Design review of the part built by this model. Coordinates are the model's own, in mm. A direction names the side the tool comes from. Coordinates: 2 decimals unless noted, no trailing zeros. Loops run counter-clockwise (first coordinate to the right, second up) from the corner with the lowest first, then second, coordinate; pieces in that order, holes last.
Q1. Add section B-B on z = 19.5. Give the boundary of the cut face in (x, y).
Q2. Wall thickness on probe 1 along Y at (x, z) = (26.5, 10.5); probe 2 along X at (y, z) = (-26.5, 14); probe 3 along Y at (x, z) = (-19, 2): over which ranges is each line inside the solid? List them lowest first.
Q3. Add section A-A on y = 26. Give the boundary of the cut face in (x, z).
Q4. Draft analysis for pull direction X (two halves, no side actions). For faces 3 (the face through (-23.38, -6.41, 12.52)), 4 (the face through (-1, 1, 25.4)), state which applies: released by +X, released by -X, zero draft, split by the parting line, or undercut.
Q5. Machinability: for faces 1 (the face through (17.24, -17.04, 12.52)), 2 (the face through (-1, 1, 0)), which of the approach directions +Z, -Z, +X, -X, +Y, -Y give a long, thin tool a straight path to every point of the face, cutting with its end or side? Answer none if there is none.
Q6. Add section D-D on y = -30. Give the boundary of the cut face in (x, z), and give its area (3 significant figures).
Q7. Add section C-C on x = 2. Give the boundary of the cut face in (y, z), and give its area (3 significant figures).
Q8. For P1, Ø5, axis at x = 20, z = 8, coming from the -Y side; P2, Ø10, axis at y = 16.5, z = 7.5, coming from the -X side; P3, Ø1.5, axis at y = 26, z = 9, coming from the +X side, all flat-tipped, find the tip position at first contact; note any pin that passes through.
```python
from build123d import *

# Parameters (mm, degrees)
F0_R     = 12.7
F1_DEPTH = 25.4


with BuildPart() as f1:
    # F0 (on Top) → F1 (new body)
    with BuildSketch(Plane.XY):
        with BuildLine():
            Line((7.3707728384, 23.1299660417), (4.863097807, 23.7839000386))
            ThreePointArc((4.863097807, 23.7839000386), (-4.0567226722, 14.7436122877), (-16.3457517616, 17.9482595445))
            Line((-16.3457517616, 17.9482595445), (-18.165912731, 16.1035162613))
            ThreePointArc((-18.165912731, 16.1035162613), (-15.3688283269, 11.9626305103), (-14.3857332102, 7.0632285104))
            ThreePointArc((-14.3857332102, 7.0632285104), (-16.9842741732, -0.6342077722), (-23.7165246, -5.1817064972))
            Line((-23.7165246, -5.1817064972), (-23.029010538, -7.6803837773))
            ThreePointArc((-23.029010538, -7.6803837773), (-11.9623656452, -9.823859748), (-6.9598019278, -19.9253187849))
            ThreePointArc((-6.9598019278, -19.9253187849), (-7.0629636452, -21.5407646313), (-7.3707728384, -23.1299660417))
            Line((-7.3707728384, -23.1299660417), (-4.863097807, -23.7839000386))
            ThreePointArc((-4.863097807, -23.7839000386), (4.0567226722, -14.7436122877), (16.3457517616, -17.9482595445))
            Line((16.3457517616, -17.9482595445), (18.165912731, -16.1035162613))
            ThreePointArc((18.165912731, -16.1035162613), (14.7967041208, -3.8585812536), (23.7165246, 5.1817064972))
            Line((23.7165246, 5.1817064972), (23.029010538, 7.6803837773))
            ThreePointArc((23.029010538, 7.6803837773), (10.7399814486, 10.8850310341), (7.3707728384, 23.1299660417))
        make_face()
        Circle(F0_R, mode=Mode.SUBTRACT)
        Circle(F0_R)
        with BuildLine():
            ThreePointArc((39.7857332102, -7.0632285104), (34.7831694928, 3.0382305265), (23.7165246, 5.1817064972))
            Line((23.7165246, 5.1817064972), (27.0857332102, -7.0632285104))
            Line((27.0857332102, -7.0632285104), (18.165912731, -16.1035162613))
            ThreePointArc((18.165912731, -16.1035162613), (31.9851352101, -18.7801333936), (39.7857332102, -7.0632285104))
        make_face()
        with BuildLine():
            ThreePointArc((20.1259312823, -26.9885472953), (19.1428361656, -22.0891452954), (16.3457517616, -17.9482595445))
            Line((16.3457517616, -17.9482595445), (7.4259312823, -26.9885472953))
            Line((7.4259312823, -26.9885472953), (-4.863097807, -23.7839000386))
            ThreePointArc((-4.863097807, -23.7839000386), (5.810485436, -39.5853855779), (20.1259312823, -26.9885472953))
        make_face()
        with BuildLine():
            Line((-27.0857332102, 7.0632285104), (-18.165912731, 16.1035162613))
            ThreePointArc((-18.165912731, 16.1035162613), (-39.3747622996, 10.2678757672), (-23.7165246, -5.1817064972))
            Line((-23.7165246, -5.1817064972), (-27.0857332102, 7.0632285104))
        make_face()
        with BuildLine():
            ThreePointArc((32.3598019278, 19.9253187849), (21.2752477741, 32.5221570675), (7.3707728384, 23.1299660417))
            Line((7.3707728384, 23.1299660417), (19.6598019278, 19.9253187849))
            Line((19.6598019278, 19.9253187849), (23.029010538, 7.6803837773))
            ThreePointArc((23.029010538, 7.6803837773), (29.7612609647, 12.2278825023), (32.3598019278, 19.9253187849))
        make_face()
        with BuildLine():
            Line((-16.3457517616, 17.9482595445), (-7.4259312823, 26.9885472953))
            Line((-7.4259312823, 26.9885472953), (4.863097807, 23.7839000386))
            ThreePointArc((4.863097807, 23.7839000386), (5.1709070002, 25.373101449), (5.2740687177, 26.9885472953))
            ThreePointArc((5.2740687177, 26.9885472953), (-12.3253332823, 38.7054521786), (-16.3457517616, 17.9482595445))
        make_face()
        with BuildLine():
            Line((-19.6598019278, -19.9253187849), (-23.029010538, -7.6803837773))
            ThreePointArc((-23.029010538, -7.6803837773), (-28.579622407, -28.9656065358), (-7.3707728384, -23.1299660417))
            Line((-7.3707728384, -23.1299660417), (-19.6598019278, -19.9253187849))
        make_face()
        with BuildLine():
            Line((4.863097807, 23.7839000386), (-7.4259312823, 26.9885472953))
            Line((-7.4259312823, 26.9885472953), (-16.3457517616, 17.9482595445))
            ThreePointArc((-16.3457517616, 17.9482595445), (-4.0567226722, 14.7436122877), (4.863097807, 23.7839000386))
        make_face()
        with BuildLine():
            Line((27.0857332102, -7.0632285104), (23.7165246, 5.1817064972))
            ThreePointArc((23.7165246, 5.1817064972), (14.7967041208, -3.8585812536), (18.165912731, -16.1035162613))
            Line((18.165912731, -16.1035162613), (27.0857332102, -7.0632285104))
        make_face()
        with BuildLine():
            Line((19.6598019278, 19.9253187849), (7.3707728384, 23.1299660417))
            ThreePointArc((7.3707728384, 23.1299660417), (10.7399814486, 10.8850310341), (23.029010538, 7.6803837773))
            Line((23.029010538, 7.6803837773), (19.6598019278, 19.9253187849))
        make_face()
        with BuildLine():
            ThreePointArc((-14.3857332102, 7.0632285104), (-15.3688283269, 11.9626305103), (-18.165912731, 16.1035162613))
            Line((-18.165912731, 16.1035162613), (-27.0857332102, 7.0632285104))
            Line((-27.0857332102, 7.0632285104), (-23.7165246, -5.1817064972))
            ThreePointArc((-23.7165246, -5.1817064972), (-16.9842741732, -0.6342077722), (-14.3857332102, 7.0632285104))
        make_face()
        with BuildLine():
            ThreePointArc((-6.9598019278, -19.9253187849), (-11.9623656452, -9.823859748), (-23.029010538, -7.6803837773))
            Line((-23.029010538, -7.6803837773), (-19.6598019278, -19.9253187849))
            Line((-19.6598019278, -19.9253187849), (-7.3707728384, -23.1299660417))
            ThreePointArc((-7.3707728384, -23.1299660417), (-7.0629636452, -21.5407646313), (-6.9598019278, -19.9253187849))
        make_face()
        with BuildLine():
            Line((7.4259312823, -26.9885472953), (16.3457517616, -17.9482595445))
            ThreePointArc((16.3457517616, -17.9482595445), (4.0567226722, -14.7436122877), (-4.863097807, -23.7839000386))
            Line((-4.863097807, -23.7839000386), (7.4259312823, -26.9885472953))
        make_face()
    extrude(amount=F1_DEPTH)


solid = f1.part
```
Entries:
1. outline: (-23.72, -5.18) - (-23.03, -7.68) arc R12.7 ccw (long way) to (-7.37, -23.13) - (-4.86, -23.78) arc R12.7 ccw (long way) to (16.35, -17.95) - (18.17, -16.1) arc R12.7 ccw (long way) to (23.72, 5.18) - (23.03, 7.68) arc R12.7 ccw (long way) to (7.37, 23.13) - (4.86, 23.78) arc R12.7 ccw (long way) to (-16.35, 17.95) - (-18.17, 16.1) arc R12.7 ccw (long way) to start
2. probe 1: y = -19.75 to 5.62, 9.22 to 30.63
2. probe 2: x = -30.53 to -8.79, -5.26 to 20.12
2. probe 3: y = -32.61 to 16.86, 21.76 to 32.22
3. outline: (-20.09, 0) - (5.24, 0) - (5.24, 25.4) - (-20.09, 25.4) - close; (8.51, 0) - (30.81, 0) - (30.81, 25.4) - (8.51, 25.4) - close
4. face 3: undercut
4. face 4: zero draft
5. face 1: +Z, -Z
5. face 2: -Z, +X, -X, +Y, -Y
6. outline: (-27.39, 0) - (-11.93, 0) - (-11.93, 25.4) - (-27.39, 25.4) - close; (-4.91, 0) - (19.76, 0) - (19.76, 25.4) - (-4.91, 25.4) - close
6. area: 1,020 mm2
7. outline: (-38.47, 0) - (35.5, 0) - (35.5, 25.4) - (-38.47, 25.4) - close
7. area: 1,880 mm2
8. P1: stops at y = -34.72
8. P2: stops at x = -38.99
8. P3: stops at x = 31.19
